Verification items for the finished model (mm, model axes). A direction names the side the tool comes from. Give positions to 0.01 mm unless a question says otherwise; leave off trailing zeros. Write each loop counter-clockwise with the first axis right and the second up, starting at its lowest first coordinate (ties: lowest second). Pieces come first, ordered by that corner, then holes.
from build123d import *

# Parameters (mm, degrees)
SKETCH1_W          = 19.05
SKETCH1_H          = 31.75
EXTRUDE1_DEPTH     = 1.5875
SKETCH3_R          = 3.571875
CUT_EXTRUDE6_DEPTH = 25.989408261
SKETCH5_R          = 3.571875
CUT_EXTRUDE8_DEPTH = 25.989408261
CIRPATTERN1_COUNT  = 2
SKETCH6_W          = 7.14375
SKETCH6_H          = 4.699
CUT_EXTRUDE9_DEPTH = 25.989408261
CIRPATTERN2_COUNT  = 2


with BuildPart() as part:
    # Sketch1 → Extrude1 (new body)
    with BuildSketch(Plane(origin=(0, 0, 0), x_dir=(1, 0, 0), z_dir=(0, 1, 0))):
        with Locations((3.175, 5.588)):
            Rectangle(SKETCH1_W, SKETCH1_H)
    extrude(amount=EXTRUDE1_DEPTH)

    # Sketch3 → Cut-Extrude6 (cut, through all)
    with BuildSketch(Plane(origin=(0, 0, 0), x_dir=(1, 0, 0), z_dir=(0, 1, 0))):
        with Locations(Location((3.175, 5.588, 0), (0, 0, 270))):
            Circle(SKETCH3_R)
    extrude(amount=CUT_EXTRUDE6_DEPTH, mode=Mode.SUBTRACT)

    # Sketch5 → Cut-Extrude8 (cut, through all)
    with BuildSketch(Plane(origin=(0, 0, 0), x_dir=(1, 0, 0), z_dir=(0, 1, 0))):
        with Locations(Location((3.175, 16.764, 0), (0, 0, 270))):
            Circle(SKETCH5_R)
    cut_extrude8 = extrude(amount=CUT_EXTRUDE8_DEPTH, mode=Mode.SUBTRACT)

    # CirPattern1: Cut-Extrude8 ×2 about axis
    cirpattern1_axis = Axis((3.175, 0, -5.588), (0, 1, 0))
    for i in range(1, CIRPATTERN1_COUNT):
        add(cut_extrude8.rotate(cirpattern1_axis, i * 360 / CIRPATTERN1_COUNT), mode=Mode.SUBTRACT)

    # Sketch6 → Cut-Extrude9 (cut, through all)
    with BuildSketch(Plane(origin=(0, 0, 0), x_dir=(1, 0, 0), z_dir=(0, 1, 0))):
        with Locations((3.175, -7.9375)):
            Rectangle(SKETCH6_W, SKETCH6_H)
    cut_extrude9 = extrude(amount=CUT_EXTRUDE9_DEPTH, mode=Mode.SUBTRACT)

    # CirPattern2: Cut-Extrude9 ×2 about axis
    cirpattern2_axis = Axis((3.175, 1.5875, -5.588), (0, -1, 0))
    for i in range(1, CIRPATTERN2_COUNT):
        add(cut_extrude9.rotate(cirpattern2_axis, i * 360 / CIRPATTERN2_COUNT), mode=Mode.SUBTRACT)


solid = part.part
Item 1: Release check for a two-part mould opening along X. For faces 4 (the face through (6.747, 1, -19)), 5 (the face through (-6.35, 1, -5)), 6 (the face through (3.04, 0, -9.34)), 7 (the face through (3.096, 0.783, -13.193)) record: released by +X, released by -X, zero draft, split by the parting line, or undercut.
Answer key:
face 4: undercut
face 5: released by -X
face 6: zero draft
face 7: undercut
Item 2: Scan lines: line 1 along X through (y, z) = (0.85, -17.5); line 2 along X through (y, z) = (1.2, -3); line 3 along Z through (x, y) = (0.5, 1.15) (3 decimals). Record each from-to range of solid material in increasing order.
Answer key:
line 1: x = -6.35 to -0.4, 6.75 to 12.7
line 2: x = -6.35 to 0.71, 5.64 to 12.7
line 3: z = -14.397 to -7.955, -3.221 to 3.221
Item 3: Sectioned sample at C-C on y = 1.25. Record the cut outline in (x, z) (3 decimals), then the cut area to 3 significant figures.
Answer key:
outline: (-6.35, -21.463) - (-0.397, -21.463) - (-0.397, -16.764) arc R3.572 cw to (6.747, -16.764) - (6.747, -21.463) - (12.7, -21.463) - (12.7, 10.287) - (6.747, 10.287) - (6.747, 5.588) arc R3.572 cw to (-0.397, 5.588) - (-0.397, 10.287) - (-6.35, 10.287) - close; hole circle Ø7.144 at (3.175, -5.588)
area: 458 mm2
Item 4: Set-up check for faces 1 (the face through (12.7, 1, -5)), 2 (the face through (-0.397, 1, 8)), 3 (the face through (-0.397, 1, -19)): record each of +Z, -Z, +X, -X, +Y, -Y from which the full face is reachable in a straight line by a thin tool's end or side.
Answer key:
face 1: +Z, -Z, +X, +Y, -Y
face 2: +Z, +Y, -Y
face 3: -Z, +Y, -Y
Item 5: Sectioned sample at A-A on z = 8.5. Record the cut outline in (x, y).
Answer key:
outline: (-6.35, 0) - (-0.4, 0) - (-0.4, 1.59) - (-6.35, 1.59) - close; (6.75, 0) - (12.7, 0) - (12.7, 1.59) - (6.75, 1.59) - close
Item 6: Sectioned sample at B-B on x = 4. Record the cut outline in (y, z), then the cut area to 3 significant figures.
Answer key:
outline: (0, -13.29) - (1.59, -13.29) - (1.59, -9.06) - (0, -9.06) - close; (0, -2.11) - (1.59, -2.11) - (1.59, 2.11) - (0, 2.11) - close
area: 13.4 mm2
